```python
from build123d import *

# Parameters (mm, degrees)
SISTEMA_START              = -68.082035122
SISTEMA_ESTRUCTURAL2_DEPTH = 100
CORTAR_EXTRUIR1_REACH      = 77.896
CROQUIS9_R                 = 4


# Read off the part's stored shape, not the designer's step: Sistema estructural2
with BuildPart() as part:
    # Sistema estructural2 outline → Sistema estructural2 (new body)
    with BuildSketch(Plane.XY.offset(SISTEMA_START)):
        with BuildLine():
            ThreePointArc((15, 9.8), (13.476955262, 13.476955262), (9.8, 15))
            Line((9.8, 15), (-9.8, 15))
            ThreePointArc((-9.8, 15), (-13.476955262, 13.476955262), (-15, 9.8))
            Line((-15, 9.8), (-15, -9.8))
            ThreePointArc((-15, -9.8), (-13.476955262, -13.476955262), (-9.8, -15))
            Line((-9.8, -15), (9.8, -15))
            ThreePointArc((9.8, -15), (13.476955262, -13.476955262), (15, -9.8))
            Line((15, -9.8), (15, 9.8))
        make_face()
        with BuildLine():
            ThreePointArc((12.4, -9.8), (11.638477631, -11.638477631), (9.8, -12.4))
            Line((9.8, -12.4), (-9.8, -12.4))
            ThreePointArc((-9.8, -12.4), (-11.638477631, -11.638477631), (-12.4, -9.8))
            Line((-12.4, -9.8), (-12.4, 9.8))
            ThreePointArc((-12.4, 9.8), (-11.638477631, 11.638477631), (-9.8, 12.4))
            Line((-9.8, 12.4), (9.8, 12.4))
            ThreePointArc((9.8, 12.4), (11.638477631, 11.638477631), (12.4, 9.8))
            Line((12.4, 9.8), (12.4, -9.8))
        make_face(mode=Mode.SUBTRACT)
    extrude(amount=SISTEMA_ESTRUCTURAL2_DEPTH)

    # Cortar-Extruir1: up to this face of the body (flat: up to its plane)
    cortar_extruir1_end = Plane(part.part.faces().sort_by_distance((0, -15, -18.082035122))[0])
    # Croquis9 → Cortar-Extruir1 (cut, up to the picked face)
    with BuildSketch(Plane(origin=(0, 15, 0), x_dir=(1, 0, 0), z_dir=(0, 1, 0)), mode=Mode.PRIVATE) as cortar_extruir1_sk1:
        with Locations(Location((0, -23.532428894, 0), (0, 0, 270))):
            Circle(CROQUIS9_R)
    cortar_extruir1_tool1 = split(extrude(cortar_extruir1_sk1.sketch, amount=-CORTAR_EXTRUIR1_REACH, mode=Mode.PRIVATE), bisect_by=cortar_extruir1_end, keep=Keep.BOTH, mode=Mode.PRIVATE)
    add(cortar_extruir1_tool1.solids().sort_by(Axis((0, 15, 23.532429), (0, -1, 0)))[0], mode=Mode.SUBTRACT)


solid = part.part
```
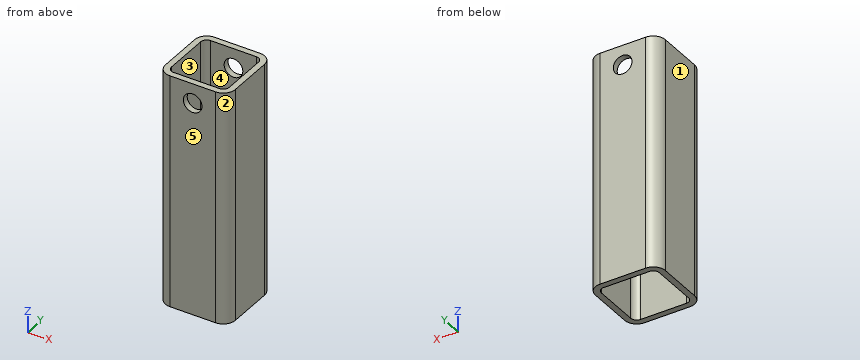
Part model, mm, in its own coordinate system. Face numbers are marked on the shaded views. A direction names the side the tool comes from. Give positions to 0.01 mm unless a question says otherwise; leave off trailing zeros. Loops run counter-clockwise (first coordinate to the right, second up) from the corner with the lowest first, then second, coordinate; pieces in that order, holes last. Notation, with made-up numbers: M -27,21 L 7,21 A15 ccw 7,26 Z; hole C -28.75,64.5 d11. An arc over 180 degrees is marked long. Return JSON: item names as keys, results as strings.
1) 3-axis set-ups, long thin cutter, end or side, ignore diameter. For the marked faces 4 and 5: which of +Z, -Z, +X, -X, +Y, -Y reach the whole face in a straight line?
Calculated:
{"face 4": "+Z, -Z", "face 5": "+Z, -Z, +X, -X, -Y"}
2) Saw through at A-A, the plane x = 7.5. List the corners of the cut face in (y, z).
Calculated:
{"outline": "M -15,-68.08 L -12.4,-68.08 L -12.4,31.92 L -15,31.92 Z; M 12.4,-68.08 L 15,-68.08 L 15,31.92 L 12.4,31.92 Z"}
3) Drill centre lines: line 1 (Y direction, x = -3.25, z = -56.5); line 2 (X direction, y = 12, z = -36). Where is each one in solid material? Low to high.
Calculated:
{"line 1": "y = -15 to -12.4, 12.4 to 15", "line 2": "x = -14.51 to -11.19, 11.19 to 14.51"}
4) Saw through at D-D, the plane z = -17. List the corners of the cut face in (x, y), then the cut area to 3 significant figures.
Calculated:
{"outline": "M -15,-9.8 A5.2 ccw -9.8,-15 L 9.8,-15 A5.2 ccw 15,-9.8 L 15,9.8 A5.2 ccw 9.8,15 L -9.8,15 A5.2 ccw -15,9.8 Z; hole M -12.4,-9.8 A2.6 ccw -9.8,-12.4 L 9.8,-12.4 A2.6 ccw 12.4,-9.8 L 12.4,9.8 A2.6 ccw 9.8,12.4 L -9.8,12.4 A2.6 ccw -12.4,9.8 Z", "area": "268 mm2"}
5) Pull direction X, two halves, no side cores. Call the marked faces 1, 2 and 3: released by +X, released by -X, zero draft, split by the parting line, or undercut.
Calculated:
{"face 1": "released by -X", "face 2": "released by +X", "face 3": "undercut"}
6) Saw through at B-B, the plane x = 0. List the corners of the cut face in (y, z).
Calculated:
{"outline": "M -15,-68.08 L -12.4,-68.08 L -12.4,19.53 L -15,19.53 Z; M -15,27.53 L -12.4,27.53 L -12.4,31.92 L -15,31.92 Z; M 12.4,-68.08 L 15,-68.08 L 15,19.53 L 12.4,19.53 Z; M 12.4,27.53 L 15,27.53 L 15,31.92 L 12.4,31.92 Z"}
